Check sheet for the modelled part. Datum: model origin and axes. Units: mm. Give positions to 0.01 mm unless a question says otherwise; leave off trailing zeros. Order: outer loops, then holes, each group sorted by start corner. A loop starts at its lowest first (then second) coordinate and runs counter-clockwise, first axis right, second up. Notation, with made-up numbers: (-18.75, 21) -> (19.25, 21) arc R23 cw to (19.25, 50) -> close; hole circle Ø8 at (76, 62). An arc over 180 degrees is marked (long way). Answer in a Markdown table with one row per item. Add a question column.
(1) Thickness scan on L1, parallel to Y at x = 4.5, z = 1.8; L2, parallel to X at y = 3, z = 0.3. Record the ranges inside material, lowest first. Write a range as [from, to].
(2) Cross-section at A-A (x = 1.5). Record the cut outline in (y, z).
(3) Cross-section at C-C (z = 2.5). Record the cut outline in (x, y), then the cut area to 3 significant figures.
(4) Cross-section at B-B (y = 8). Record the cut outline in (x, z).
(5) Go/stop test with flat-tipped pins: pin 1 (2 mm diameter, centred on x = 14.5, z = 3.5, fed in from +Y); pin 2 (1 mm diameter, centred on y = -14.5, z = 3, fed in from -X); pin 3 (2.5 mm diameter, centred on x = 11.49, y = 17.51, fed in from +Z); pin 4 (3 mm diameter, centred on x = 9, z = 2, fed in from -Y). Record where each tip stops, or that it passes through.
(6) Cross-section at D-D (y = -0.5). Record the cut outline in (x, z).
(7) Release check for a two-part mould opening along X. For faces 1 (the face through (8, 0, 5)), 2 (the face through (18.433, -10.208, 2.465)), 3 (the face through (10.06, -17.56, 2.46)) record: released by +X, released by -X, zero draft, split by the parting line, or undercut.
Autodesk Inventor part; units mm, degrees
ref_plane "YZ Plane" through (0, 0, 0) normal (1, 0, 0) x (0, 1, 0)
ref_plane "XZ Plane" through (0, 0, 0) normal (0, 1, 0) x (-1, 0, 0)
ref_plane "XY Plane" through (0, 0, 0) normal (0, 0, 1) x (1, 0, 0)
sketch "Sketch1" plane through (0, 0, 0) normal (0, 0, 1) x (1, 0, 0)
  circle A0 centre (11.5096, -17.4937) radius 1.45
  circle A1 centre (11.4904, 17.5063) radius 1.45
  line L0 (-6.5054, 9.9465) -> (-6.4946, -9.9535)
  line L1 (-6.4946, -9.9535) -> (6.5054, -9.9465)
  line L2 (6.5054, -9.9465) -> (6.4946, 9.9535)
  line L3 (6.4946, 9.9535) -> (-6.5054, 9.9465)
  arc A2 (8.0096, -17.4956) -> (11.0077, -14.0299) centre (11.5096, -17.4937) ccw
  line L4 (8.0096, -17.4956) -> (-13.9904, -17.5076)
  line L5 (-13.9904, -17.5076) -> (-14.0096, 17.4924)
  line L6 (-14.0096, 17.4924) -> (7.9904, 17.5044)
  arc A3 (10.9923, 14.0419) -> (7.9904, 17.5044) centre (11.4904, 17.5063) ccw
  line L7 (10.9923, 14.0419) -> (11.0077, -14.0299)
  ellipse E0 centre (120.0743, 0.0597) end of major axis (125.4052, -3.3899) minor radius 6.3497
  circle A4 centre (18, 0.0098) radius 1.45
  line L8 (7.9904, 17.5044) -> (8.0096, -17.4956)
  circle A5 centre (18, 0.0098) radius 4.45
  line L9 (14.8825, 18.3689) -> (22.0821, 1.7816)
  line L10 (14.8825, -18.4283) -> (22.0851, -1.7549)
  point P0 (0, 0)
  dimension "d0" = 2.9
  dimension "d1" = 3
  dimension "d2" = 7
extrude "Extrusion1" add sketch "Sketch1" along normal blind 5 contours L8 A3 L7 A2 | L4 L5 L6 L8 | A2 L7 A3 L9 A5 L10 | A5
properties part number "03_OTmic_belt_gear"
Answer below:
| question | item | result |
|---|---|---|
| 1 | L1 | y = [-17.5, -9.95], [9.95, 17.5] |
| 1 | L2 | x = [-14, -6.5], [6.5, 21.55] |
| 2 | outline | (-17.5, 0) -> (-9.95, 0) -> (-9.95, 5) -> (-17.5, 5) -> close; (9.95, 0) -> (17.5, 0) -> (17.5, 5) -> (9.95, 5) -> close |
| 3 | outline | (-14.01, 17.49) -> (-13.99, -17.51) -> (8.01, -17.5) arc R3.5 ccw to (14.88, -18.43) -> (22.09, -1.75) arc R4.45 ccw to (22.08, 1.78) -> (14.88, 18.37) arc R3.5 ccw to (7.99, 17.5) -> close; hole (-6.51, 9.95) -> (-6.49, -9.95) -> (6.51, -9.95) -> (6.49, 9.95) -> close; hole circle Ø2.9 at (11.49, 17.51); hole circle Ø2.9 at (11.51, -17.49); hole circle Ø2.9 at (18, 0.01) |
| 3 | area | 917 mm² |
| 4 | outline | (-14, 0) -> (-6.5, 0) -> (-6.5, 5) -> (-14, 5) -> close; (6.5, 0) -> (19.38, 0) -> (19.38, 5) -> (6.5, 5) -> close |
| 5 | pin 1 | stops at y = 20.37 |
| 5 | pin 2 | stops at x = -13.99 |
| 5 | pin 3 | passes through |
| 5 | pin 4 | stops at y = -20.84 |
| 6 | outline | (-14, 0) -> (-6.5, 0) -> (-6.5, 5) -> (-14, 5) -> close; (6.5, 0) -> (16.64, 0) -> (16.64, 5) -> (6.5, 5) -> close; (19.36, 0) -> (22.42, 0) -> (22.42, 5) -> (19.36, 5) -> close |
| 7 | face 1 | zero draft |
| 7 | face 2 | released by +X |
| 7 | face 3 | undercut |
